from build123d import *

# Parameters (mm, degrees)
SKETCH1_W                     = 131
SKETCH1_H                     = 124.9
SKETCH1_W_2                   = 124.6
SKETCH1_H_2                   = 118.5
BOSS_EXTRUDE1_DEPTH           = 2.4
SKETCH1_3_W                   = 131
SKETCH1_3_H                   = 124.9
SKETCH1_3_W_2                 = 124.6
SKETCH1_3_H_2                 = 118.5
BOSS_EXTRUDE2_DEPTH           = 80
CUT_EXTRUDE1_DEPTH            = 197.769729517
CUT_EXTRUDE2_REACH            = 199.577
SKETCH3_W                     = 124.6
SKETCH3_H                     = 3.362002976
SKETCH4_W                     = 129
SKETCH4_H                     = 72.65
CUT_EXTRUDE3_DEPTH            = 3.2
SKETCH5_W                     = 129
SKETCH5_H                     = 96.155451154
CUT_EXTRUDE4_DEPTH            = 2.4
FILLET1_R                     = 3
SKETCH7_R                     = 15
BOSS_EXTRUDE3_DEPTH           = 1.8
BOSS_EXTRUDE3_DRAFT           = 60
SKETCH7_R_2                   = 7.5
BOSS_EXTRUDE3_PROFILE_2_DEPTH = 1.8
BOSS_EXTRUDE3_PROFILE_2_DRAFT = 60
SKETCH6_W                     = 11.9888
SKETCH6_H                     = 2.519598063
SKETCH6_R                     = 2.5
CUT_EXTRUDE6_DEPTH            = 196.787767749


with BuildPart() as part:
    # Sketch1 → Boss-Extrude1 (new body)
    # profile 1 of 2: a face of its own
    with BuildSketch(Plane(origin=(0, 0, 0), x_dir=(1, 0, 0), z_dir=(0, 1, 0))):
        with Locations((62.3, 60.66509434)):
            Rectangle(SKETCH1_W, SKETCH1_H)
        with Locations((62.3, 60.66509434)):
            Rectangle(SKETCH1_W_2, SKETCH1_H_2, mode=Mode.SUBTRACT)
    # profile 2 of 2: a face of its own
    with BuildSketch(Plane(origin=(0, 0, 0), x_dir=(1, 0, 0), z_dir=(0, 1, 0))):
        with Locations((62.3, 60.66509434)):
            Rectangle(SKETCH1_W_2, SKETCH1_H_2)
    extrude(amount=-BOSS_EXTRUDE1_DEPTH)

    # Sketch1<3> → Boss-Extrude2 (add)
    with BuildSketch(Plane(origin=(0, 0, 0), x_dir=(1, 0, 0), z_dir=(0, 1, 0))):
        with Locations((62.3, 60.66509434)):
            Rectangle(SKETCH1_3_W, SKETCH1_3_H)
        with Locations((62.3, 60.66509434)):
            Rectangle(SKETCH1_3_W_2, SKETCH1_3_H_2, mode=Mode.SUBTRACT)
    extrude(amount=BOSS_EXTRUDE2_DEPTH)

    # Sketch2 → Cut-Extrude1 (cut, through all)
    with BuildSketch(Plane(origin=(127.8, 0, 0), x_dir=(0, 0, -1), z_dir=(1, 0, 0))):
        Polygon((-1.78490566, 13.018733893), (25.959643186, 80), (-1.78490566, 80), align=None)
    extrude(amount=-CUT_EXTRUDE1_DEPTH, mode=Mode.SUBTRACT)

    # Sketch3 → Cut-Extrude2 (cut, up to next)
    with BuildSketch(Plane(origin=(0, 2.537608886, 6.126329787), x_dir=(1, 0, 0), z_dir=(0, 0.38268343236508395, 0.9238795325112892)), mode=Mode.PRIVATE) as cut_extrude2_sk1:
        with Locations((62.3, 18.025689446)):
            Rectangle(SKETCH3_W, SKETCH3_H)
    cut_extrude2_tool1 = extrude(cut_extrude2_sk1.sketch, amount=-CUT_EXTRUDE2_REACH, mode=Mode.PRIVATE) & part.part
    add(cut_extrude2_tool1.solids().sort_by_distance((62.3, 19.191174, -0.771803))[0], mode=Mode.SUBTRACT)

    # Sketch4 → Cut-Extrude3 (cut)
    with BuildSketch(Plane(origin=(0, 2.537608886, 6.126329787), x_dir=(1, 0, 0), z_dir=(0, 0.38268343236508423, 0.9238795325112892))):
        with Locations((62.3, 47.519687958)):
            Rectangle(SKETCH4_W, SKETCH4_H)
    extrude(amount=-CUT_EXTRUDE3_DEPTH, mode=Mode.SUBTRACT)

    # Sketch5 → Cut-Extrude4 (cut)
    with BuildSketch(Plane(origin=(0, 80, 0), x_dir=(1, 0, 0), z_dir=(0, 1, 0))):
        with Locations((62.3, 74.037368763)):
            Rectangle(SKETCH5_W, SKETCH5_H)
    extrude(amount=-CUT_EXTRUDE4_DEPTH, mode=Mode.SUBTRACT)

    # Fillet1
    fillet1_edges = [part.edges().sort_by_distance(p)[0] for p in [
        (-2.7, 80, -25.959643186),
        (127.3, 80, -25.959643186),
    ]]
    fillet(fillet1_edges, radius=FILLET1_R)


with BuildPart() as boss_extrude3_tool:
    # Sketch7 → Boss-Extrude3 (with draft: the straight prism first)
    with BuildSketch(Plane.XY.offset(-119.91509434)):
        with Locations((40.466666667, 60)):
            Circle(SKETCH7_R)
    extrude(amount=BOSS_EXTRUDE3_DEPTH)
    # Boss-Extrude3: the draft: its side faces are tilted about the plane it starts from
    boss_extrude3_sides = [boss_extrude3_tool.faces().sort_by_distance(p)[0] for p in [
        (25.466666667, 60, -119.01509434),
    ]]
    draft(boss_extrude3_sides, Plane.XY.offset(-119.91509434), BOSS_EXTRUDE3_DRAFT)


with BuildPart() as part_1:
    add(part.part)

    # Boss-Extrude3: add boss_extrude3_tool
    add(boss_extrude3_tool.part)


with BuildPart() as boss_extrude3_profile_2_tool:
    # Sketch7 → Boss-Extrude3 profile 2 (with draft: the straight prism first)
    with BuildSketch(Plane.XY.offset(-119.91509434)):
        with Locations((84.133333333, 60)):
            Circle(SKETCH7_R_2)
    extrude(amount=BOSS_EXTRUDE3_PROFILE_2_DEPTH)
    # Boss-Extrude3 profile 2: the draft: its side faces are tilted about the plane it starts from
    boss_extrude3_profile_2_sides = [boss_extrude3_profile_2_tool.faces().sort_by_distance(p)[0] for p in [
        (76.633333333, 60, -119.01509434),
    ]]
    draft(boss_extrude3_profile_2_sides, Plane.XY.offset(-119.91509434), BOSS_EXTRUDE3_PROFILE_2_DRAFT)


with BuildPart() as part_2:
    add(part_1.part)

    # Boss-Extrude3 profile 2: add boss_extrude3_profile_2_tool
    add(boss_extrude3_profile_2_tool.part)

    # Sketch6 → Cut-Extrude6 (cut, through all)
    with BuildSketch(Plane(origin=(0, 0, -123.11509434), x_dir=(-1, 0, 0), z_dir=(0, 0, -1))):
        with BuildLine():
            Line((-34.472266667, 57.480401937), (-46.461066667, 57.480401937))
            ThreePointArc((-46.461066667, 57.480401937), (-40.466666667, 53.4976), (-34.472266667, 57.480401937))
        make_face()
        with Locations((-40.466666667, 58.740200969)):
            Rectangle(SKETCH6_W, SKETCH6_H)
        with Locations((-40.466666667, 61.259799032)):
            Rectangle(SKETCH6_W, SKETCH6_H)
        with BuildLine():
            ThreePointArc((-34.472266667, 62.519598063), (-40.466666667, 66.5024), (-46.461066667, 62.519598063))
            Line((-46.461066667, 62.519598063), (-34.472266667, 62.519598063))
        make_face()
        with Locations((-84.133333333, 60)):
            Circle(SKETCH6_R)
    extrude(amount=-CUT_EXTRUDE6_DEPTH, mode=Mode.SUBTRACT)


solid = part_2.part
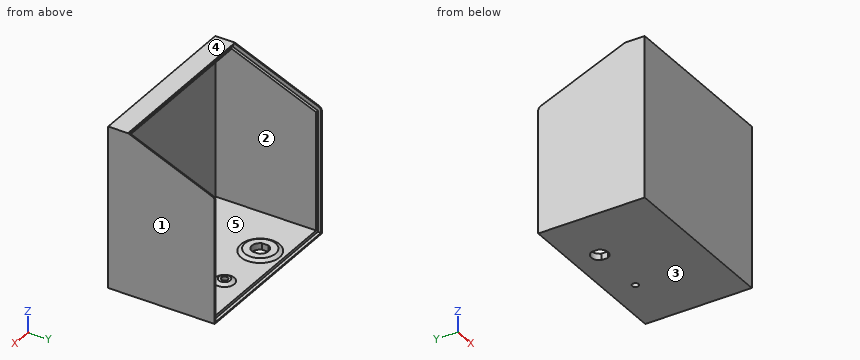
Model file for the job. Use its own axes, mm. Face numbers are marked on the shaded views. A direction names the side the tool comes from. Give positions to 0.01 mm unless a question says otherwise; leave off trailing zeros. Order: outer loops, then holes, each group sorted by start corner. A loop starts at its lowest first (then second) coordinate and runs counter-clockwise, first axis right, second up. Notation, with made-up numbers: (35.5, 84.25) - (46.5, 84.25) arc R18 cw to (46.5, 90.25) - close; hole circle Ø2 at (77.25, -12). An arc over 180 degrees is marked (long way). Write item = value, one per line. Start each with the question number.
1. Cut at A-A, the plane x = 119. List the corners of the cut face in (y, z).
2. Probe line 1 along X through (y, z) = (35, -101); line 2 along Z through (x, y) = (48.5, 6); line 3 along Y through (x, z) = (45, -60). List the from-to ranges inside material, lowest first.
3. Two-plate mould, pull along Z, no slides. Class the marked faces 3, 4 and 5: pulls with the +Z half, pulls with the -Z half, needs draft (parallel to the pull), parting line crosses it, or undercut.
4. Which spindle directions (+Z, -Z, +X, -X, +Y, -Y) get a long thin tool onto all of the face, cutting with end or side? Do the marked faces 1 and 2. Say none if no direction does.
5. Drop flat-ended pins along their axis: P1, Ø4, axis at x = 96.5, z = -63, coming from the +Y side; P2, Ø12, axis at x = 92.5, y = 60.5, coming from the +Z side; P3, Ø0.7, axis at x = 31, y = 78.5, coming from the +Z side. Give the stop position or say it passes through.
6. Cut at B-B, the plane z = -46. List the corners of the cut face in (x, y).
7. Cut at D-D, the plane y = 60. List the corners of the cut face in (x, z).
8. Cut at C-C, the plane y = 37. List the corners of the cut face in (x, z), and give its area (3 significant figures).
Taken from the geometry:
q1.outline = (-2.4, -123.12) - (80, -123.12) - (80, -122.12) - (77.6, -122.12) - (77.6, -119.92) - (0, -119.92) - (0, -1.42) - (12.38, -1.42) - (11.66, -1.11) - (12.86, 1.78) - (-2.4, 1.78) - close
q2.line_1 = -3.2 to 0, 124.6 to 127.8
q2.line_2 = -123.12 to -119.92, -1.42 to 1.78
q2.line_3 = -2.4 to 0
q3.face_3 = pulls with the -Z half
q3.face_4 = pulls with the +Z half
q3.face_5 = undercut
q4.face_1 = +Z, -Z, +X, +Y, -Y
q4.face_2 = +Y
q5.P1 = 0
q5.P2 = -118.12
q5.P3 = -122.12
q6.outline = (-3.2, -2.4) - (127.8, -2.4) - (127.8, 80) - (126.8, 80) - (126.8, 77.6) - (124.6, 77.6) - (124.6, 0) - (0, 0) - (0, 77.6) - (-2.2, 77.6) - (-2.2, 80) - (-3.2, 80) - close
q7.outline = (-3.2, -123.12) - (34.47, -123.12) - (34.47, -118.12) - (28.58, -118.12) - (25.47, -119.92) - (0, -119.92) - (0, -21.14) - (-2.2, -21.14) - (-2.2, -17.68) - (-3.2, -17.68) - close; (46.46, -123.12) - (81.63, -123.12) - (81.63, -118.12) - (79.75, -118.12) - (76.63, -119.92) - (55.47, -119.92) - (52.35, -118.12) - (46.46, -118.12) - close; (86.63, -123.12) - (127.8, -123.12) - (127.8, -17.68) - (126.8, -17.68) - (126.8, -21.14) - (124.6, -21.14) - (124.6, -119.92) - (91.63, -119.92) - (88.52, -118.12) - (86.63, -118.12) - close
q8.outline = (-3.2, -123.12) - (127.8, -123.12) - (127.8, -8.15) - (126.8, -8.15) - (126.8, -11.61) - (124.6, -11.61) - (124.6, -119.92) - (0, -119.92) - (0, -11.61) - (-2.2, -11.61) - (-2.2, -8.15) - (-3.2, -8.15) - close
q8.area = 1,120 mm²
